Autodesk Inventor part; units mm, degrees
ref_plane "YZ Plane" through (0, 0, 0) normal (1, 0, 0) x (0, 1, 0)
ref_plane "XZ Plane" through (0, 0, 0) normal (0, 1, 0) x (-1, 0, 0)
ref_plane "XY Plane" through (0, 0, 0) normal (0, 0, 1) x (1, 0, 0)
sketch "Skizze1" plane through (0, 0, 0) normal (0, 0, 1) x (1, 0, 0)
  line L0 (-31.2875, 34) -> (31.2875, 34)
  line L1 (31.2875, 34) -> (31.2875, -34)
  line L2 (31.2875, -34) -> (-31.2875, -34)
  line L3 (-31.2875, -34) -> (-31.2875, 34)
  point P0 (0, 0)
  dimension "d0" = 62.575
  dimension "d1" = 68
  dimension "d40" = 31.2875
  dimension "d41" = 34
extrude "Extrusion1" add sketch "Skizze1" along normal blind 6
sketch "Skizze2" plane through (0, 0, 0) normal (0, 0, -1) x (-1, 0, 0)
  line L0 (31.2875, 34) -> (31.2875, -34)
  point P0 (18.7125, -12)
  point P1 (-21.2875, -12)
  point P2 (0, 0)
  point P3 (-21.2875, 12)
  point P4 (18.7125, 12)
  point P5 (-21.2875, -12)
  dimension "d9" = 40
  dimension "d10" = 12.575
  dimension "d20" = 24
  dimension "d21" = 12
hole "Bohrung1" at (-18.7125, -12, 0) at (21.2875, -12, 0) at (21.2875, 12, 0) at (-18.7125, 12, 0) direction (0, 0, 1) diameter 4.5 end through all counterbore diameter 8 counterbore depth 4
sketch "Skizze3" plane through (0, 0, 6) normal (0, 0, 1) x (1, 0, 0)
  circle A0 centre (21.2875, -12) radius 2.25
  circle A1 centre (-18.7125, -12) radius 2.25
  circle A2 centre (-18.7125, 12) radius 2.25
  circle A3 centre (21.2875, 12) radius 2.25
  point P0 (0, 0)
  point P1 (0, -12)
  point P2 (0, 12)
hole "Bohrung2" at (0, -12, 6) at (0, 12, 6) direction (0, 0, -1) diameter 5 depth 2
sketch "Skizze4" plane through (0, 0, 6) normal (0, 0, 1) x (1, 0, 0)
  line L0 (-31.2875, -34) -> (31.2875, -34)
  line L1 (31.2875, 34) -> (-31.2875, 34)
  line L2 (-31.2875, 34) -> (-31.2875, -34)
  point P0 (0, 0)
  point P1 (-16.2875, -25)
  point P2 (-16.2875, 25)
  dimension "d29" = 9
  dimension "d30" = 9
  dimension "d31" = 15
hole "Bohrung3" at (-16.2875, -25, 6) at (-16.2875, 25, 6) direction (0, 0, -1) diameter 6.6 end through all
sketch "Skizze5" plane through (0, 0, 6) normal (0, 0, 1) x (1, 0, 0)
  line L0 (-31.2875, -34) -> (31.2875, -34)
  line L1 (31.2875, -34) -> (31.2875, 34)
  line L2 (-1.2875, -34) -> (31.2875, -34)
  line L3 (31.2875, -34) -> (31.2875, -20)
  line L4 (31.2875, -20) -> (3.7125, -20)
  line L5 (-1.2875, -25) -> (-1.2875, -34)
  line L6 (-1.2875, 34) -> (31.2875, 34)
  line L7 (31.2875, 34) -> (31.2875, 20)
  line L8 (31.2875, 20) -> (3.7125, 20)
  line L9 (-1.2875, 25) -> (-1.2875, 34)
  line L10 (-31.2875, 34) -> (-31.2875, -34)
  line L11 (31.2875, 34) -> (-31.2875, 34)
  arc A0 (3.7125, -20) -> (-1.2875, -25) centre (3.7125, -25) ccw
  arc A1 (-1.2875, 25) -> (3.7125, 20) centre (3.7125, 25) ccw
  point P0 (0, 0)
  point P1 (-1.2875, -29.5)
  dimension "d42" = 40
  dimension "d43" = 20
  dimension "d44" = 30
  dimension "d45" = 30
  dimension "d46" = 5
extrude "Extrusion2" cut sketch "Skizze5" against normal through all contours L5 A0 L4 L1 L0 | L6 L1 L8 A1 L9
properties part number "TS_Halterung_Fuehrungszylinder_int"
CAD build for the part. Positions are in the model's coordinates, mm. A direction names the side the tool comes from. Give positions to 0.01 mm unless a question says otherwise; leave off trailing zeros. Loops run counter-clockwise (first coordinate to the right, second up) from the corner with the lowest first, then second, coordinate; pieces in that order, holes last. Notation, with made-up numbers: (4.5, 62) - (50.5, 62) arc R19 cw to (50.5, 92) - close; hole circle Ø3 at (23.25, 50.25). An arc over 180 degrees is marked (long way). Put each result on its own line as item: value.
Q1. Slice it at D-D (x = 1). Give the cut face in (y, z).
Filled in:
outline: (-20.8, 0) - (20.8, 0) - (20.8, 6) - (14.29, 6) - (14.29, 4) - (9.71, 4) - (9.71, 6) - (-9.71, 6) - (-9.71, 4) - (-14.29, 4) - (-14.29, 6) - (-20.8, 6) - close
Q2. Slice it at A-A (y = -12). Give the cut face in (x, z).
Filled in:
outline: (-31.29, 0) - (-22.71, 0) - (-22.71, 4) - (-20.96, 4) - (-20.96, 6) - (-31.29, 6) - close; (-16.46, 4) - (-14.71, 4) - (-14.71, 0) - (17.29, 0) - (17.29, 4) - (19.04, 4) - (19.04, 6) - (2.5, 6) - (2.5, 4) - (-2.5, 4) - (-2.5, 6) - (-16.46, 6) - close; (23.54, 4) - (25.29, 4) - (25.29, 0) - (31.29, 0) - (31.29, 6) - (23.54, 6) - close
Q3. Mould opens along X. For faces 4 (the face through (-7, 0, 6)), 5 (the face through (-17, -10, 4)), 6 (the face through (0.216, -21.426, 3.042)) say: pulls with the +X half, pulls with the -X half, needs draft (parallel to the pull), parting line crosses it, or undercut.
Filled in:
face 4: needs draft
face 5: undercut
face 6: pulls with the +X half
Q4. Flat gauge pins, fed straight in: pin 1 (2.5 mm diameter, centred on x = 21.29, y = 12, fed in from -Z); pin 2 (1.8 mm diameter, centred on x = 15, z = 2.5, fed in from +Y); pin 3 (3 mm diameter, centred on y = -30, z = 3.5, fed in from +X); pin 4 (2.5 mm diameter, centred on x = 23, y = -11, fed in from -Z). Where does each tip first touch, or does it go through?
Filled in:
pin 1: passes through
pin 2: stops at y = 20
pin 3: stops at x = -1.29
pin 4: stops at z = 4
Q5. Slice it at C-C (z = 5.15). Give the number of separate pieces and of enclosed holes in the cut face, plus the area to 3 significant figures.
Filled in:
separate pieces: 1
enclosed holes: 8
area: 3,180 mm²
Q6. Slice it at B-B (y = 23.5). Give the cut face in (x, z).
Filled in:
outline: (-31.29, 0) - (-19.23, 0) - (-19.23, 6) - (-31.29, 6) - close; (-13.35, 0) - (-1.06, 0) - (-1.06, 6) - (-13.35, 6) - close
Q7. Tool access for faces 1 (the face through (-1.288, 29, 3)), 2 (the face through (-0.1, -9.5, 5)), 3 (the face through (-22.68, 11.48, 2.03)): list every direction of +Z, -Z, +X, -X, +Y, -Y with a clear straight run to the whole face (end or side of a thin tool).
Filled in:
face 1: +Z, -Z, +X, +Y
face 2: +Z
face 3: -Z
Q8. Probe line 1 along X through (y, z) = (-12, 1.1); line 2 along X through (y, z) = (12, 5.3); line 3 along Y through (x, z) = (21.5, 3.25). List the from-to ranges inside material, lowest first.
Filled in:
line 1: x = -31.29 to -22.71, -14.71 to 17.29, 25.29 to 31.29
line 2: x = -31.29 to -20.96, -16.46 to -2.5, 2.5 to 19.04, 23.54 to 31.29
line 3: y = -20 to -15.99, -8.01 to 8.01, 15.99 to 20
